Source: three-view drawing plus pictorial views. Frame: mm from the lowest corner of the part. A direction names the side the tool comes from. Give positions to 0.01 mm unless a question says otherwise; leave off trailing zeros. Write each loop counter-clockwise with the first axis right and the second up, starting at its lowest first coordinate (ties: lowest second). Pieces come first, ordered by that corner, then holes. Notation, with made-up numbers: M -2,48.5 L 46,48.5 A27 ccw 46,68.5 Z; hole C 65,43.25 d10. An arc over 180 degrees is marked long. One line per question, with ' | ' between items.
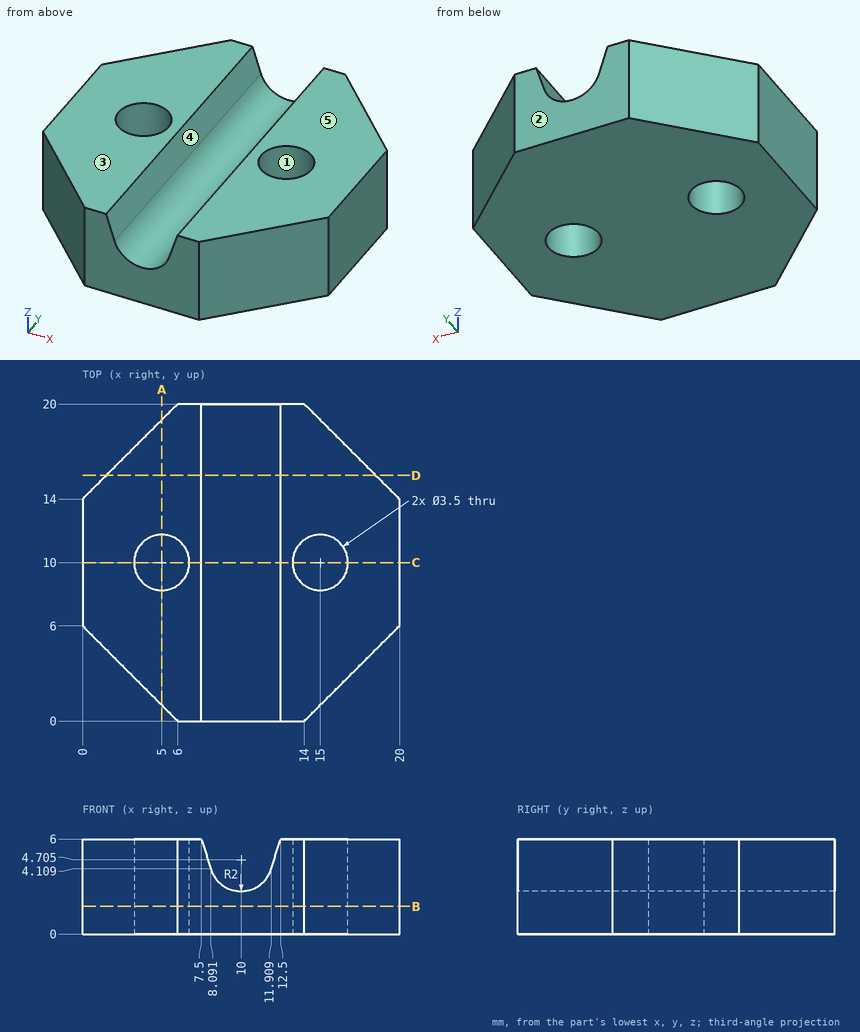
(1) Material intervals for L1, parallel to X at y = 10.75, z = 3.25; L2, parallel to X at y = 8.75, z = 0.5 (1 decimal); L3, parallel to Y at x = 4, z = 1.75 (1 decimal), sorted ascending. Write a range as [from, to].
Working result:
L1: x = [0, 3.42], [6.58, 8.63], [11.37, 13.42], [16.58, 20] | L2: x = [0, 3.8], [6.2, 13.8], [16.2, 20] | L3: y = [2, 8.6], [11.4, 18]
(2) Cut plane B-B, the plane z = 1.75. Return loops of the section in (x, y).
Working result:
outline: M 0,6 L 6,0 L 14,0 L 20,6 L 20,14 L 14,20 L 6,20 L 0,14 Z; hole C 5,10 d3.5; hole C 15,10 d3.5
(3) Cut plane D-D, the plane y = 15.5. Return loops of the section in (x, z) (1 decimal).
Working result:
outline: M 1.5,0 L 18.5,0 L 18.5,6 L 12.5,6 L 11.9,4.1 A2 cw 8.1,4.1 L 7.5,6 L 1.5,6 Z
(4) Set-up query: the marked faces 4 and 5. Return all of +Z, -Z, +X, -X, +Y, -Y with unobstructed straight access to the full face (end or side cutting, diameter ignored); none if empty.
Working result:
face 4: +Z, +Y, -Y | face 5: +Z, +X, -X, +Y, -Y
(5) First-contact query: P1, Ø2, axis at y = 16, z = 4, coming from the -X side. Flat tip, straight axial feed; report the tip coordinate or a pass-through.
Working result:
P1: stops at x = 1
(6) Cut plane C-C, the plane y = 10. Count the separate pieces of the cut face and the enclosed holes in it.
Working result:
separate pieces: 3 | enclosed holes: 0
(7) Cut plane A-A, the plane x = 5. Return loops of the section in (y, z).
Working result:
outline: M 1,0 L 8.25,0 L 8.25,6 L 1,6 Z; M 11.75,0 L 19,0 L 19,6 L 11.75,6 Z
(8) Draft query along Y for the marked faces 1, 2 and 3. Return one class per face: released by +Y, released by -Y, zero draft, split by the parting line, or undercut.
Working result:
face 1: undercut | face 2: released by +Y | face 3: zero draft
